Model file for the job. Use its own axes, mm. A direction names the side the tool comes from. Coordinates: 2 decimals unless noted, no trailing zeros. Order: outer loops, then holes, each group sorted by start corner. A loop starts at its lowest first (then second) coordinate and runs counter-clockwise, first axis right, second up. Notation, with made-up numbers: M 32.25,13.5 L 50.25,13.5 A13 cw 50.25,31.5 Z; hole C 84,-3 d3. An arc over 180 degrees is marked long. Return JSON: item names as keys, results as strings.
Autodesk Inventor part; units mm, degrees
ref_plane "YZ Plane" through (0, 0, 0) normal (1, 0, 0) x (0, 1, 0)
ref_plane "XZ Plane" through (0, 0, 0) normal (0, 1, 0) x (-1, 0, 0)
ref_plane "XY Plane" through (0, 0, 0) normal (0, 0, 1) x (1, 0, 0)
sketch "Sketch1" plane through (0, 0, 0) normal (0, 1, 0) x (-1, 0, 0)
  circle A0 centre (0, 0) radius 6
  circle A1 centre (0, 0) radius 4.5
  dimension "d2" = 12
  dimension "d3" = 9
extrude "Extrusion1" add sketch "Sketch1" along normal blind 8
sketch "Sketch2" plane through (0, 8, 0) normal (0, 1, 0) x (1, 0, 0)
  circle A0 centre (0, 0) radius 8.5
  circle A1 centre (0, 0) radius 4.5
  dimension "d6" = 17
extrude "Extrusion2" add sketch "Sketch2" along normal blind 4
sketch "Sketch3" plane through (0, 12, 0) normal (0, 1, 0) x (1, 0, 0)
  line L0 (0, 0) -> (-10, 0)
  line L1 (-10, 5.7735) -> (0, 11.547)
  line L2 (0, 11.547) -> (10, 5.7735)
  line L3 (10, 5.7735) -> (10, -5.7735)
  line L4 (10, -5.7735) -> (0, -11.547)
  line L5 (0, -11.547) -> (-10, -5.7735)
  line L6 (-10, -5.7735) -> (-10, 5.7735)
  circle A0 centre (0, 0) radius 6
  dimension "d9" = 10
extrude "Extrusion3" add sketch "Sketch3" along normal blind 10
sketch "Sketch4" plane through (0, 22, 0) normal (0, 1, 0) x (1, 0, 0)
  circle A0 centre (0, 0) radius 9
  circle A1 centre (0, 0) radius 6.5
  dimension "d12" = 18
  dimension "d13" = 13
extrude "Extrusion4" add sketch "Sketch4" along normal blind 2
sketch "Sketch5" plane through (0, 24, 0) normal (0, 1, 0) x (1, 0, 0)
  circle A0 centre (0, 0) radius 6.5
  circle A1 centre (0, 0) radius 6.5
  circle A2 centre (0, 0) radius 7.5
  dimension "d16" = 15
extrude "Extrusion5" add sketch "Sketch5" along normal blind 1.5
fillet "Fillet1" radius 1.5 1 edges at (-7.5, 24, 0)
sketch "Sketch6" plane through (0, 25.5, 0) normal (0, 1, 0) x (1, 0, 0)
  circle A0 centre (0, 0) radius 7.5
  circle A1 centre (0, 0) radius 6.5
extrude "Extrusion6" cut sketch "Sketch6" against normal blind 13.5 contours A1
thread "Thread1"
sketch "Sketch7" plane through (0, 25.5, 0) normal (0, 1, 0) x (1, 0, 0)
  circle A0 centre (0, 0) radius 6.5
properties part number "entrada_manguera_alicat_flujo"
Item 1: 3-axis set-ups, long thin cutter, end or side, ignore diameter. For faces 1 (the cylindrical face through (4.57, 9.972, 7.167)), 2 (the flat face through (10, 17, 0)), 3 (the flat face through (-1.54, 12, -4.42)): which of +Z, -Z, +X, -X, +Y, -Y reach the whole face in a straight line?
Check result:
{"face 1": "-Y", "face 2": "+Z, -Z, +X, +Y, -Y", "face 3": "+Y"}
Item 2: Saw through at C-C (z = -10). Write the cut outline in (x, y), and give its area (3 significant figures).
Check result:
{"outline": "M -2.68,12 L 2.68,12 L 2.68,22 L -2.68,22 Z", "area": "53.6 mm2"}
Item 3: Drop a flat-ended pin along its axis: pin 1 Ø2 at (x, y) = (-4, 16.5) entering from -Z. Give the stop position or say it passes through.
Check result:
{"pin 1": "stops at z = -9.81"}
Item 4: Saw through at D-D (y = 2.5). Write the cut outline in (x, z), and give its area (3 significant figures).
Check result:
{"outline": "C 0,0 d12; hole C 0,0 d9", "area": "49.5 mm2"}
Item 5: Pull direction Z, two halves, no side cores. Call faces 4 (the cylindrical face through (-5.158, 18.844, 3.955)), 5 (the flat face through (-6, 25.5, -3)), 6 (the cylindrical face through (-1.172, 22.986, 8.923)): +Z half, -Z half, draft (parallel to the pull), parting line (faces both ways), or undercut.
Check result:
{"face 4": "undercut", "face 5": "draft", "face 6": "parting line"}
Item 6: Saw through at B-B (y = 22.75). Write the cut outline in (x, z).
Check result:
{"outline": "C 0,0 d18; hole C 0,0 d13"}
Item 7: Wall check: line 1 (X direction, y = 15.5, z = 0); line 2 (X direction, y = 16.25, z = 3); line 3 (Z direction, x = 0, y = 3.25). Give the ranges that are in metal, low to high.
Check result:
{"line 1": "x = -10 to -6.5, 6.5 to 10", "line 2": "x = -10 to -5.77, 5.77 to 10", "line 3": "z = -6 to -4.5, 4.5 to 6"}
Item 8: Saw through at A-A (y = 19.75). Write the cut outline in (x, z), and give its area (3 significant figures).
Check result:
{"outline": "M -10,-5.77 L 0,-11.55 L 10,-5.77 L 10,5.77 L 0,11.55 L -10,5.77 Z; hole C 0,0 d13", "area": "214 mm2"}
